Study the drawing (mm; zero at the part's minimum x, y, z) and answer. Round coordinates to 2 decimals unless told otherwise and drop trailing zeros. Write each loop counter-clockwise with the first axis right and the second up, starting at its lowest first coordinate (ties: lowest second). Pieces come first, ordered by that corner, then holes.
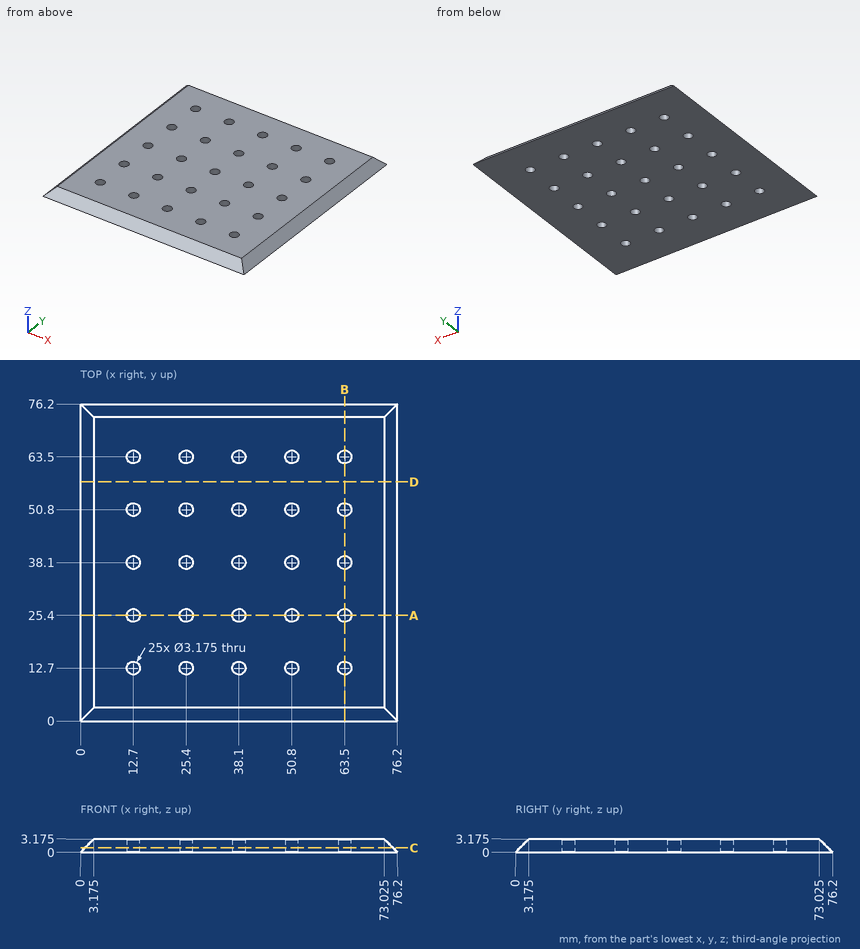
Q1. Find section D-D (y = 57.5). Determine the outline of the cut face in (x, z) (3 decimals), plus the area to 3 significant figures.
Q2. Given pin 1 (3 mm diameter, centred on x = 38.1, y = 12.7, fed in from +Z); pin 2 (1.5 mm diameter, centred on y = 31.5, z = 0.5, fed in from +X); pin 3 (1 mm diameter, centred on x = 58.5, z = 1, fed in from -Y), each flat-ended and moving along its own axis, determine where each tip first touches the part or whether it passes through.
Q3. Find section A-A (y = 25.4). Determine the outline of the cut face in (x, z) (1 decimal), plus the area to 3 significant figures.
Q4. Find the intervals of material crossed by L1, parallel to Y at x = 25.4, z = 1.85; L2, parallel to X at y = 38.1, z = 2.4, in increasing order.
Q5. Find section C-C (z = 1.05). Count the separate pieces of the cut face and the enclosed holes in it, plus the area to 3 significant figures.
Report:
1. outline: (0, 0) - (76.2, 0) - (73.025, 3.175) - (3.175, 3.175) - close
1. area: 232 mm2
2. pin 1: passes through
2. pin 2: stops at x = 76.2
2. pin 3: stops at y = 0.5
3. outline: (0, 0) - (11.1, 0) - (11.1, 3.2) - (3.2, 3.2) - close; (14.3, 0) - (23.8, 0) - (23.8, 3.2) - (14.3, 3.2) - close; (27, 0) - (36.5, 0) - (36.5, 3.2) - (27, 3.2) - close; (39.7, 0) - (49.2, 0) - (49.2, 3.2) - (39.7, 3.2) - close; (52.4, 0) - (61.9, 0) - (61.9, 3.2) - (52.4, 3.2) - close; (65.1, 0) - (76.2, 0) - (73, 3.2) - (65.1, 3.2) - close
3. area: 181 mm2
4. L1: y = 1.85 to 11.11, 14.29 to 23.81, 26.99 to 36.51, 39.69 to 49.21, 52.39 to 61.91, 65.09 to 74.35
4. L2: x = 2.4 to 11.11, 14.29 to 23.81, 26.99 to 36.51, 39.69 to 49.21, 52.39 to 61.91, 65.09 to 73.8
5. separate pieces: 1
5. enclosed holes: 25
5. area: 5,290 mm2
